Autodesk Inventor part; units mm, degrees
ref_plane "YZ Plane" through (0, 0, 0) normal (1, 0, 0) x (0, 1, 0)
ref_plane "XZ Plane" through (0, 0, 0) normal (0, 1, 0) x (-1, 0, 0)
ref_plane "XY Plane" through (0, 0, 0) normal (0, 0, 1) x (1, 0, 0)
sketch "Block1" plane through (0, 0, 0) normal (0, 0, 1) x (1, 0, 0)
  line L0 (-105.9874, 13.2259) -> (-105.9874, 0.5259)
  line L1 (109.9126, 13.2259) -> (-105.9874, 13.2259)
  line L2 (109.9126, 0.5259) -> (109.9126, 13.2259)
  line L3 (86.6216, -12.9211) -> (-82.6964, -12.9211)
  line L4 (-105.9874, 0.5259) -> (-82.6964, -12.9211)
  line L5 (109.9126, 0.5259) -> (86.6216, -12.9211)
  circle A0 centre (-99.6374, 9.7141) radius 2.0955
  circle A1 centre (103.5626, 9.7141) radius 2.0955
  point P0 (3.9065, 11.282)
  dimension "d30" = 4.191
  dimension "d31" = 4.191
sketch "Sketch1" plane through (0, 0, 0) normal (0, 0, 1) x (1, 0, 0)
  line L0 (-6.35, -6.35) -> (-6.35, -19.05)
  line L1 (209.55, -6.35) -> (-6.35, -6.35)
  line L2 (209.55, -19.05) -> (209.55, -6.35)
  line L3 (186.259, -32.4971) -> (16.941, -32.4971)
  line L4 (-6.35, -19.05) -> (16.941, -32.4971)
  line L5 (209.55, -19.05) -> (186.259, -32.4971)
  circle A0 centre (0, -9.8618) radius 2.0955
  circle A1 centre (203.2, -9.8618) radius 2.0955
  point P0 (0, 0)
extrude "Extrusion1" add sketch "Sketch1" along normal blind 1.5875
feature "Bend Part1" [suppressed]
equation "\"BendRadius\" = Thickness"
equation "\"BendReliefWidth\" = Thickness"
equation "\"BendReliefDepth\" = 0.5 * Thickness"
equation "\"CornerReliefSize\" = 4 * Thickness"
equation "\"MinimumRemnant\" = 2 * Thickness"
equation "\"TransitionRadius\" = BendRadius"
equation "\"JacobiRadiusSize\" = BendRadius"
equation "\"GapSize\" = Thickness"
properties part number "wedge" material "Acetal Resin, White"
Geometry check sheet. Reference: the model listing, model coordinates, mm. Give positions to 0.01 mm unless a question says otherwise; leave off trailing zeros. Order: outer loops, then holes, each group sorted by start corner. A loop starts at its lowest first (then second) coordinate and runs counter-clockwise, first axis right, second up. Notation, with made-up numbers: (-39, -29.75) -> (-32, -29.75) arc R16 cw to (-32, -14.75) -> close; hole circle Ø10 at (-7.75, 39.25). An arc over 180 degrees is marked (long way). Write each question's results on one line, items separated by ' | '. Start each with the question number.
(1) Gauge pin test, flat end, axial feed: P1, Ø4, axis at x = 203.2, y = -9.86, coming from the +Z side. Record the tip position at first contact, or that the pin passes through.
(2) Scan lines: line 1 (X direction, y = -10, z = 0.7); line 2 (Y direction, x = 0, z = 0.8); line 3 (X direction, y = -27.5, z = 1.5). Record each from-to range of solid material in increasing order.
(3) Mould release check, pull along Y, two halves, no side actions. Record for faces 1 (the face through (100, -19, 0)), 2 (the face through (-0.27, -11.94, 0.78)), 3 (the face through (204.327, -11.629, 0.783)), 4 (the face through (5.13, -25.68, 0.78)): pulls with the +Y half, pulls with the -Y half, needs draft (parallel to the pull), parting line crosses it, or undercut.
(4) Sectioned sample at A-A (z = 0.55). Enter the section's corners in (x, y).
(5) Sectioned sample at B-B (x = 203.2). Enter the section's corners in (y, z), plus the area to 3 significant figures.
(6) Sectioned sample at C-C (y = -22.5). Enter the section's corners in (x, z), plus the area to 3 significant figures.
Answer below:
1) P1: through
2) line 1: -6.35 to -2.09, 2.09 to 201.11, 205.29 to 209.55 | line 2: -22.72 to -11.96, -7.77 to -6.35 | line 3: 8.29 to 194.91
3) face 1: needs draft | face 2: undercut | face 3: undercut | face 4: pulls with the -Y half
4) outline: (-6.35, -19.05) -> (16.94, -32.5) -> (186.26, -32.5) -> (209.55, -19.05) -> (209.55, -6.35) -> (-6.35, -6.35) -> close; hole circle Ø4.19 at (0, -9.86); hole circle Ø4.19 at (203.2, -9.86)
5) outline: (-22.72, 0) -> (-11.96, 0) -> (-11.96, 1.59) -> (-22.72, 1.59) -> close; (-7.77, 0) -> (-6.35, 0) -> (-6.35, 1.59) -> (-7.77, 1.59) -> close | area: 19.3 mm2
6) outline: (-0.37, 0) -> (203.57, 0) -> (203.57, 1.59) -> (-0.37, 1.59) -> close | area: 324 mm2
